Source: three-view drawing plus pictorial views. Frame: mm from the lowest corner of the part. A direction names the side the tool comes from. Round coordinates to 2 decimals unless told otherwise and drop trailing zeros. Order: outer loops, then holes, each group sorted by start corner. A loop starts at its lowest first (then second) coordinate and runs counter-clockwise, first axis right, second up. Notation, with made-up numbers: M 5,-28 L 40,-28 A18 ccw 40,1 Z; hole C 80.25,-28.5 d3. An arc over 180 degrees is marked long. Return JSON: item names as keys, results as strings. Group by question number.
Q1. Contact query for flat-ended pins moving along their axis: pin 1 (9 mm diameter, centred on x = 26, z = 20.5, fed in from +Y); pin 2 (1 mm diameter, centred on x = 24, z = 18.5, fed in from +Y); pin 3 (2 mm diameter, centred on x = 18, y = 33, fed in from +Z). Output: stop coordinate, or through.
Q2. Access query for the marked faces 1, 2 and 3. Directions: +Z, -Z, +X, -X, +Y, -Y. A direction counts if a zero-diameter tool reaches every point of the face in a straight line with its end or side. Return the directions, or none.
Q3. Cut plane D-D on z = 46.5. Output: boundary loops of the cut face in (x, y), and give its area (3 significant figures).
Q4. Ray query, probe 1 along Z at (x, y) = (19, 19.5); probe 2 along Y at (x, z) = (22.5, 25). Return the intervals inside material, ascending.
Q5. Cut plane A-A on z = 35. Output: boundary loops of the cut face in (x, y), and give its area (3 significant figures).
Q6. Cut plane B-B on x = 20. Output: boundary loops of the cut face in (y, z), and give its area (3 significant figures).
Q7. Cut plane C-C on y = 23. Output: boundary loops of the cut face in (x, z), and give its area (3 significant figures).
Q8. Mould query, pull axis Z, two halves, no side actions, for the marked faces 4, 5 and 6. Classes: released by +Z, released by -Z, zero draft, split by the parting line, or undercut.
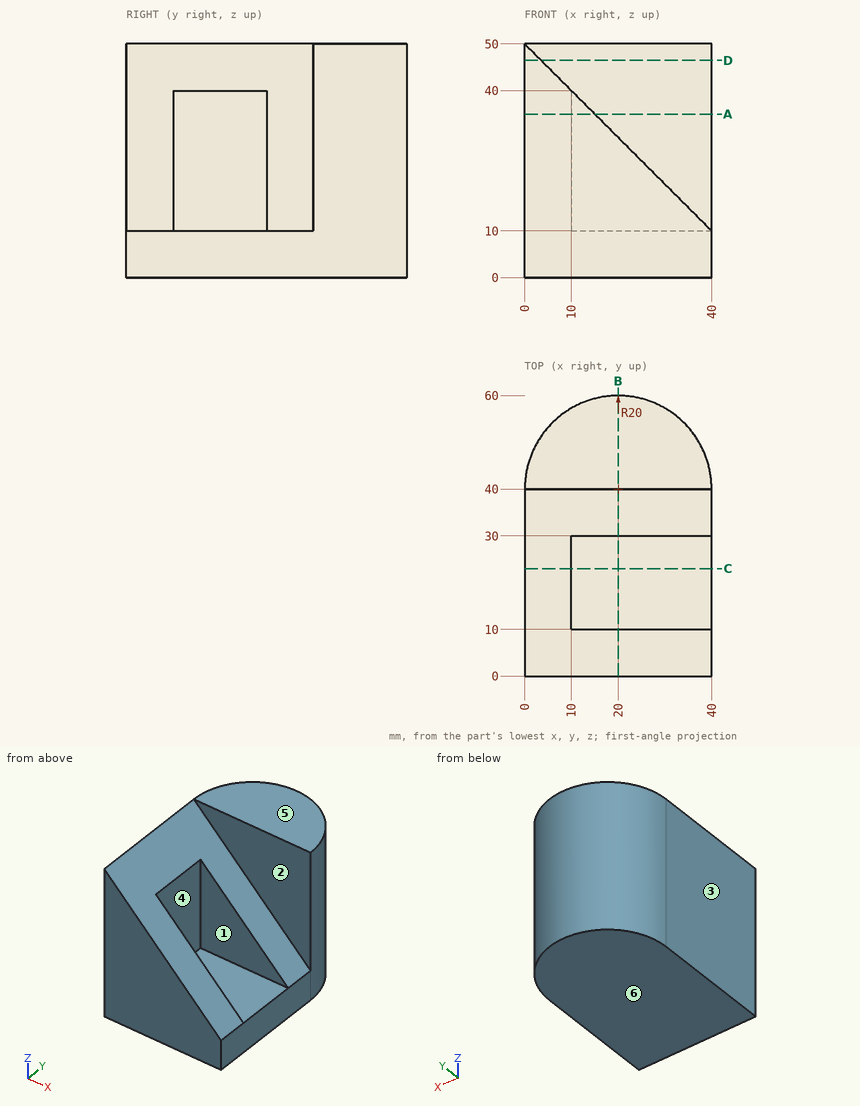
Result sheet:
{
 "1": {"pin 1": "stops at y = 59.94", "pin 2": "stops at y = 59.69", "pin 3": "stops at z = 33"},
 "2": {"face 1": "+Z, +X", "face 2": "+Z, +X, -Y", "face 3": "+Z, -Z, -X, +Y, -Y"},
 "3": {"outline": "M 0,0 L 3.5,0 L 3.5,40 L 40,40 A20 ccw 0,40 Z", "area": "768 mm²"},
 "4": {"probe 1": "z = 0 to 10", "probe 2": "y = 0 to 10, 30 to 59.84"},
 "5": {"outline": "M 0,0 L 15,0 L 15,10 L 10,10 L 10,30 L 15,30 L 15,40 L 40,40 A20 ccw 0,40 Z", "area": "1,130 mm²"},
 "6": {"outline": "M 0,0 L 60,0 L 60,50 L 40,50 L 40,30 L 30,30 L 30,10 L 10,10 L 10,30 L 0,30 Z", "area": "1,800 mm²"},
 "7": {"outline": "M 0,0 L 40,0 L 40,10 L 10,10 L 10,40 L 0,50 Z", "area": "750 mm²"},
 "8": {"face 4": "zero draft", "face 5": "released by +Z", "face 6": "released by -Z"}
}
